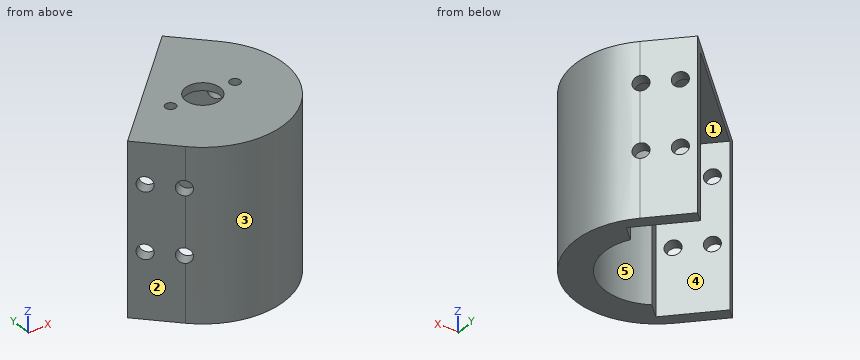
```python
from build123d import *

# Parameters (mm, degrees)
BOSS_EXTRUDE1_DEPTH = 63.5
BOSS_EXTRUDE2_START = 3
SKETCH4_R           = 6.731
SKETCH4_R_2         = 2.0309967
BOSS_EXTRUDE2_DEPTH = 3
SKETCH5_R           = 2.921
CUT_EXTRUDE3_DEPTH  = 102.608265033


with BuildPart() as part:
    # Sketch2 → Boss-Extrude1 (new body)
    with BuildSketch(Plane.XY):
        with BuildLine():
            Line((5.832216731, 32.244069222), (9.199812777, 35.611665268))
            Line((9.199812777, 35.611665268), (22.405739022, 22.405739022))
            ThreePointArc((22.405739022, 22.405739022), (22.405739022, -22.405739022), (-22.405739022, -22.405739022))
            Line((-22.405739022, -22.405739022), (-35.611665268, -9.199812777))
            Line((-35.611665268, -9.199812777), (-32.244069222, -5.832216731))
            Line((-32.244069222, -5.832216731), (-15.361187714, -22.715098239))
            Line((-15.361187714, -22.715098239), (-10.21301234, -17.566922865))
            ThreePointArc((-10.21301234, -17.566922865), (14.368409794, -14.368409794), (17.566922865, 10.21301234))
            Line((17.566922865, 10.21301234), (22.715098239, 15.361187714))
            Line((22.715098239, 15.361187714), (5.832216731, 32.244069222))
        make_face()
    extrude(amount=-BOSS_EXTRUDE1_DEPTH)

    # Sketch4 → Boss-Extrude2 (add)
    with BuildSketch(Plane.XY.offset(BOSS_EXTRUDE2_START)):
        with BuildLine():
            Line((9.199812777, 35.611665268), (-35.611665268, -9.199812777))
            Line((-35.611665268, -9.199812777), (-22.405739022, -22.405739022))
            ThreePointArc((-22.405739022, -22.405739022), (22.405739022, -22.405739022), (22.405739022, 22.405739022))
            Line((22.405739022, 22.405739022), (9.199812777, 35.611665268))
        make_face()
        Circle(SKETCH4_R, mode=Mode.SUBTRACT)
        with Locations((12.5, 0)):
            Circle(SKETCH4_R_2, mode=Mode.SUBTRACT)
        with Locations((-12.5, 0)):
            Circle(SKETCH4_R_2, mode=Mode.SUBTRACT)
    extrude(amount=-BOSS_EXTRUDE2_DEPTH)

    # Sketch5 → Cut-Extrude3 (cut, through all)
    with BuildSketch(Plane(origin=(-22.405739022, -22.405739022, 0), x_dir=(0, 0, 1), z_dir=(-0.7071067811865476, -0.7071067811865476, 0))):
        with Locations(Location((-12.7, 0.3626, 0), (0, 0, 352.869161209))):
            Circle(SKETCH5_R)
        with Locations(Location((-12.7, 13.0626, 0), (0, 0, 270))):
            Circle(SKETCH5_R)
        with Locations(Location((-38.1, 13.0626, 0), (0, 0, 270))):
            Circle(SKETCH5_R)
        with Locations(Location((-38.1, 0.3626, 0), (0, 0, 352.869161209))):
            Circle(SKETCH5_R)
    extrude(amount=-CUT_EXTRUDE3_DEPTH, mode=Mode.SUBTRACT)


solid = part.part
```
Geometry: final body of the model. Coordinates: model frame, mm. Face numbers are marked on the shaded views. A direction names the side the tool comes from. Round coordinates to 2 decimals unless told otherwise and drop trailing zeros. Write each loop counter-clockwise with the first axis right and the second up, starting at its lowest first coordinate (ties: lowest second). Pieces come first, ordered by that corner, then holes. Notation, with made-up numbers: (9.25, 32.5) -> (27.25, 32.5) arc R19 cw to (27.25, 36.5) -> close; hole circle Ø9 at (-31.75, -32). An arc over 180 degrees is marked (long way). Use CSV: the item, a comma, the result in double quotes. Start each with the question number.
Q1. First-contact query: pin 1 Ø8 at (x, z) = (-13.5, -16.5) entering from -Y; pin 2 Ø12 at (x, z) = (-13, -15) entering from -Y; pin 3 Ø3 at (x, z) = (23.5, -5) entering from +Y; pin 4 Ø3.5 at (x, y) = (-12.5, 0) entering from -Z. Flat tips, straight axial feed; report the tip coordinate or a pass-through.
Q2. Section C-C (x = 0). Return loops of the section in (y, z).
Q3. Section D-D (z = -49). Return loops of the section in (x, y).
Q4. Section B-B (y = 0). Return loops of the section in (x, z).
Q5. Pull-direction query (Y, two-part tool) for the marked faces 3, 4 and 5; classes: pulls with the +Y half, pulls with the -Y half, needs draft (parallel to the pull), parting line crosses it, or undercut.
Q6. Line query: L1, parallel to Z at x = -19.5, y = -22; L2, parallel to X at y = -21, z = -38; L3, parallel to Z at x = -10.5, y = -9.5. Output: solid intervals per line, ascending.
Q7. Section A-A (z = -11.5). Return loops of the section in (x, y), plus the area to 3 significant figures.
Q8. Reachability of the marked faces 1 and 2 from +Z, -Z, +X, -X, +Y, -Y: full face, straight path, thin tool, end or side. Return the list, or none.
Result sheet:
1,pin 1,"y = -30.23"
1,pin 2,"y = -30.9"
1,pin 3,"y = 22.81"
1,pin 4,"through"
2,outline,"(-31.69, -63.5) -> (-20.32, -63.5) -> (-20.32, 0) -> (-6.73, 0) -> (-6.73, 3) -> (-31.69, 3) -> close; (6.73, 0) -> (26.41, 0) -> (26.41, 3) -> (6.73, 3) -> close"
3,outline,"(-35.61, -9.2) -> (-22.41, -22.41) arc R31.69 ccw to (22.41, 22.41) -> (9.2, 35.61) -> (5.83, 32.24) -> (22.72, 15.36) -> (17.57, 10.21) arc R20.32 cw to (-10.21, -17.57) -> (-15.36, -22.72) -> (-32.24, -5.83) -> close"
4,outline,"(-26.41, 0) -> (-14.53, 0) -> (-14.53, 3) -> (-26.41, 3) -> close; (-10.47, 0) -> (-6.73, 0) -> (-6.73, 3) -> (-10.47, 3) -> close; (6.73, 0) -> (10.47, 0) -> (10.47, 3) -> (6.73, 3) -> close; (14.53, 0) -> (20.32, 0) -> (20.32, -63.5) -> (31.69, -63.5) -> (31.69, 3) -> (14.53, 3) -> close"
5,face 3,"parting line crosses it"
5,face 4,"pulls with the +Y half"
5,face 5,"undercut"
6,L1,"-63.5 to -40.1, -36.1 to -14.7, -10.7 to 3"
6,L2,"-17.38 to -17.08, -13.65 to 23.73"
6,L3,"0 to 3"
7,outline,"(-35.61, -9.2) -> (-33.53, -11.29) -> (-30.16, -7.92) -> (-32.24, -5.83) -> close; (-29.76, -15.05) -> (-24.55, -20.27) -> (-21.18, -16.9) -> (-26.39, -11.68) -> close; (-20.72, -23.97) arc R31.69 ccw to (23.97, 20.72) -> (20.66, 17.41) -> (22.72, 15.36) -> (17.57, 10.21) arc R20.32 cw to (-10.21, -17.57) -> (-15.36, -22.72) -> (-17.41, -20.66) -> close; (5.83, 32.24) -> (7.92, 30.16) -> (11.29, 33.53) -> (9.2, 35.61) -> close; (11.68, 26.39) -> (16.9, 21.18) -> (20.27, 24.55) -> (15.05, 29.76) -> close"
7,area,"934 mm²"
8,face 1,"-Z"
8,face 2,"+Z, -Z, -X, -Y"
